Build history of the part. All positions in model axes, mm. Coordinates: 2 decimals unless noted, no trailing zeros. Order: outer loops, then holes, each group sorted by start corner. A loop starts at its lowest first (then second) coordinate and runs counter-clockwise, first axis right, second up. Notation, with made-up numbers: (42.5, 60.5) - (47.5, 60.5) arc R12 ccw to (47.5, 71.5) - close; hole circle Ø6 at (34, 5). An arc over 180 degrees is marked (long way). One line per item, written item: value.
from build123d import *

# Parameters (mm, degrees)
F0_R     = 9.525
F0_R_2   = 3.0861
F1_DEPTH = 3.175
F2_R     = 2.9845
F3_DEPTH = 3.175


with BuildPart() as f1:
    # F0 (on Right) → F1 (new body)
    with BuildSketch(Plane.YZ):
        with BuildLine():
            Line((-102.220117, -7.91324), (-1.240234, -15.826479))
            ThreePointArc((-1.240234, -15.826479), (9.855756, -12.445067), (15.68961, -2.419045))
            ThreePointArc((15.68961, -2.419045), (15.808298, -1.453729), (15.867652, -0.482956))
            ThreePointArc((15.867652, -0.482956), (15.869841, -0.404681), (15.871644, -0.326396))
            ThreePointArc((15.871644, -0.326396), (10.897173, 11.544143), (-1.240234, 15.826479))
            Line((-1.240234, 15.826479), (-102.220117, 7.91324))
            ThreePointArc((-102.220117, 7.91324), (-109.5375, 0), (-102.220117, -7.91324))
        make_face()
        with BuildLine():
            ThreePointArc((-25.989111, 7.517578), (-17.859375, 0), (-25.989111, -7.517578))
            Line((-25.989111, -7.517578), (-82.790295, -3.06638))
            ThreePointArc((-82.790295, -3.06638), (-85.625781, 0), (-82.790295, 3.06638))
            Line((-82.790295, 3.06638), (-25.989111, 7.517578))
        make_face(mode=Mode.SUBTRACT)
        Circle(F0_R, mode=Mode.SUBTRACT)
        with Locations((-101.6, 0)):
            Circle(F0_R_2, mode=Mode.SUBTRACT)
    extrude(amount=F1_DEPTH)

    # F2 (on face) → F3 (join)
    with BuildSketch(Plane.YZ.offset(3.175)):
        with BuildLine():
            ThreePointArc((32.802387, 24.602289), (35.182837, 34.857256), (24.782335, 33.226167))
            ThreePointArc((24.782335, 33.226167), (14.335256, 20.997637), (-0.901989, 15.849355))
            ThreePointArc((-0.901989, 15.849355), (10.901756, 11.539816), (15.875, 0))
            ThreePointArc((15.875, 0), (20.515606, 14.931586), (32.802387, 24.602289))
        make_face()
        with Locations((30.532871, 30.532871)):
            Circle(F2_R, mode=Mode.SUBTRACT)
    extrude(amount=-F3_DEPTH)


solid = f1.part
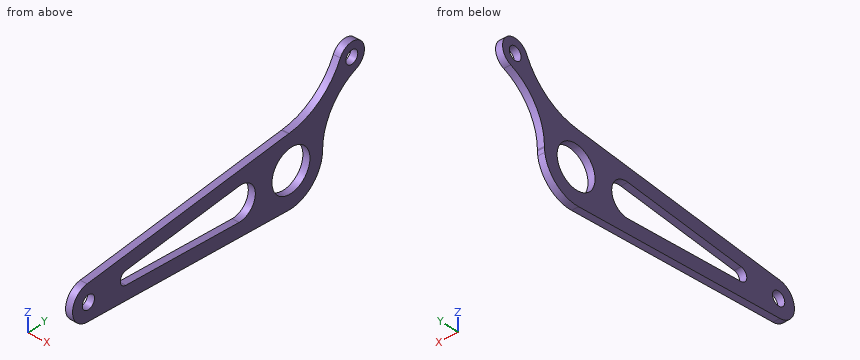
1. Band-saw the part on D-D, the plane y = -90.5. Give the cut face in (x, z) (3 decimals), and give its area (3 significant figures).
Values found:
outline: (0, -8.832) - (3.175, -8.832) - (3.175, 8.832) - (0, 8.832) - close
area: 56.1 mm2
2. Band-saw the part on A-A, the plane y = -45.5. Give the cut face in (x, z) (3 decimals).
Values found:
outline: (0, -12.358) - (3.175, -12.358) - (3.175, -5.989) - (0, -5.989) - close; (0, 5.989) - (3.175, 5.989) - (3.175, 12.358) - (0, 12.358) - close
3. Band-saw the part on B-B, the plane x = 1.7. Count the separate pieces of the cut face and the enclosed holes in it, and give its area (3 significant figures).
Values found:
separate pieces: 1
enclosed holes: 4
area: 2,220 mm2
4. Flat gauge pins, fed straight in: P1, Ø17, axis at y = 0, z = 0, coming from the +X side; P2, Ø1, axis at x = 2.5, y = -7, coming from the -Z side. Where does each tip first touch, or does it go through?
Values found:
P1: passes through
P2: stops at z = -15.41
5. Probe line 1 along Z through (x, y) = (1.65, -67.5); line 2 along Y through (x, z) = (2.2, 2); line 3 along Z through (x, y) = (0.25, -64). List the from-to ranges inside material, lowest first.
Values found:
line 1: z = -10.63 to -4.26, 4.26 to 10.63
line 2: y = -109.28 to -103.95, -99.25 to -84.89, -18.13 to -9.31, 9.31 to 15.95
line 3: z = -10.91 to -4.54, 4.54 to 10.91
6. Band-saw the part on C-C, the plane y = 3. Give the cut face in (x, z) (3 decimals), and give its area (3 significant figures).
Values found:
outline: (0, -15.589) - (3.175, -15.589) - (3.175, -9.04) - (0, -9.04) - close; (0, 9.04) - (3.175, 9.04) - (3.175, 16.327) - (0, 16.327) - close
area: 43.9 mm2
